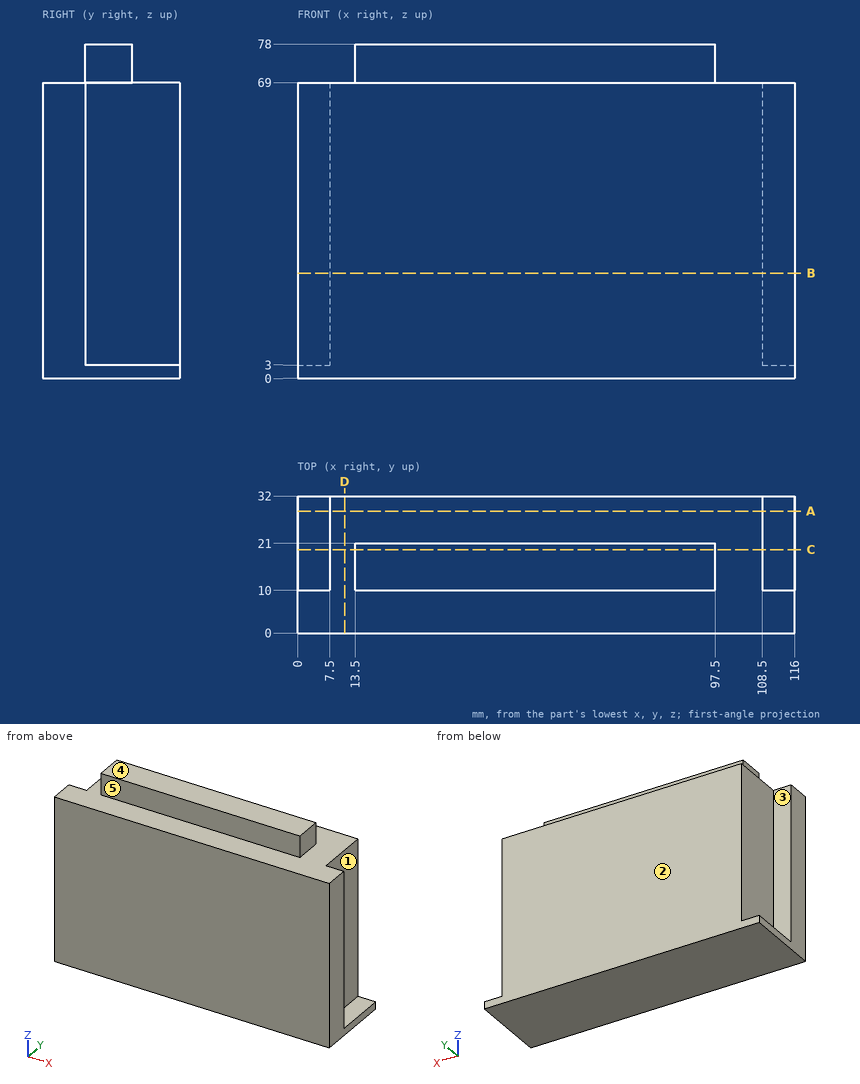
Geometry check sheet. Reference: drawing and pictorial views, mm from the part's lowest x, y, z. A direction names the side the tool comes from. Round coordinates to 2 decimals unless told otherwise and drop trailing zeros. Write each loop counter-clockwise with the first axis right and the second up, starting at its lowest first coordinate (ties: lowest second). Pieces come first, ordered by that corner, then holes.
Item 1: Section check C-C (y = 19.5). Record the boundary of the cut face in (x, z), plus the area to 3 significant figures.
Determined:
outline: (0, 0) - (116, 0) - (116, 3) - (108.5, 3) - (108.5, 69) - (97.5, 69) - (97.5, 78) - (13.5, 78) - (13.5, 69) - (7.5, 69) - (7.5, 3) - (0, 3) - close
area: 7,770 mm2
Item 2: Section check B-B (z = 24.5). Record the boundary of the cut face in (x, y), plus the area to 3 significant figures.
Determined:
outline: (0, 0) - (116, 0) - (116, 10) - (108.5, 10) - (108.5, 32) - (7.5, 32) - (7.5, 10) - (0, 10) - close
area: 3,380 mm2
Item 3: Material ranges on line 1 along Z through (x, y) = (101, 15); line 2 along X through (y, z) = (30.5, 40.5); line 3 along Z through (x, y) = (5.5, 21.5), recorded low to high.
Determined:
line 1: z = 0 to 69
line 2: x = 7.5 to 108.5
line 3: z = 0 to 3
Item 4: Go/stop test with flat-tipped pins: pin 1 Ø1 at (y, z) = (18.5, 54) entering from +X; pin 2 Ø8 at (y, z) = (16, 10) entering from -X; pin 3 Ø2 at (x, z) = (2.5, 33.5) entering from +Y. Record where each tip stops, or that it passes through.
Determined:
pin 1: stops at x = 108.5
pin 2: stops at x = 7.5
pin 3: stops at y = 10
Item 5: Access from +Z, -Z, +X, -X, +Y, -Y to the whole of each face (thin tool, end or side, straight path). Record for the marked faces 1, 2, 3, 4 and 5.
Determined:
face 1: +Z, +X, +Y
face 2: +Z, -Z, +X, -X, +Y
face 3: +Z, -X, +Y
face 4: +Z, +X, -X, +Y, -Y
face 5: +Z, +X, -X, -Y
Item 6: Section check A-A (y = 28.5). Record the boundary of the cut face in (x, z).
Determined:
outline: (0, 0) - (116, 0) - (116, 3) - (108.5, 3) - (108.5, 69) - (7.5, 69) - (7.5, 3) - (0, 3) - close
Item 7: Section check D-D (x = 11). Record the boundary of the cut face in (y, z), plus the area to 3 significant figures.
Determined:
outline: (0, 0) - (32, 0) - (32, 69) - (0, 69) - close
area: 2,210 mm2
